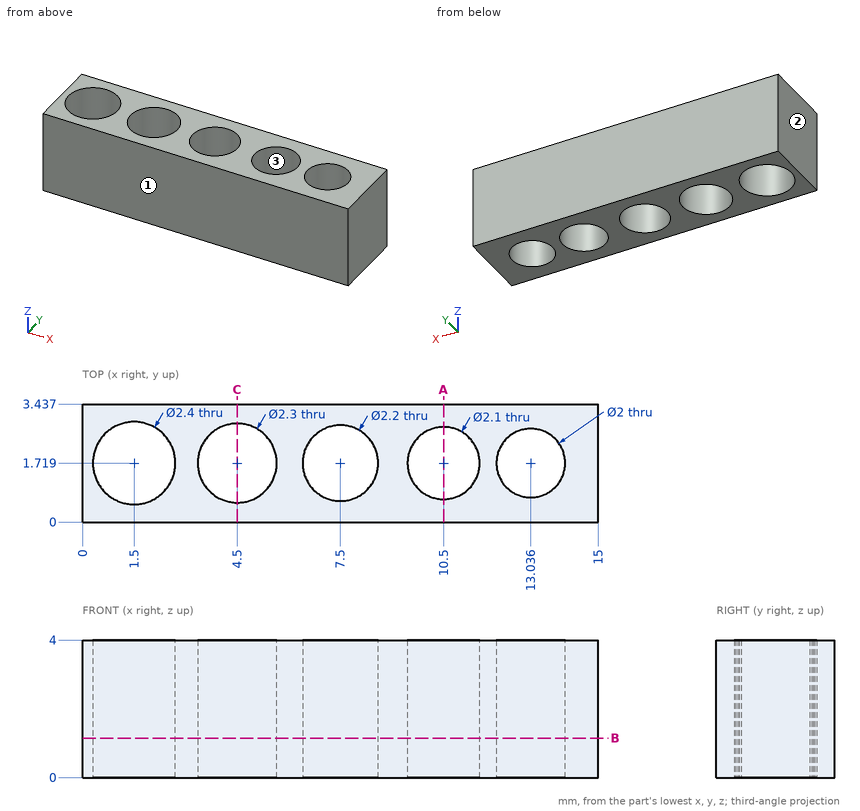
Here's the drawing with two shaded views (mm, measured from the low corner). I have some questions. Give positions to 0.01 mm unless a question says otherwise; leave off trailing zeros. Order: outer loops, then holes, each group sorted by start corner. A loop starts at its lowest first (then second) coordinate and runs counter-clockwise, first axis right, second up. Notation, with made-up numbers: (70.25, 21) -> (109.25, 21) arc R20 ccw to (109.25, 53) -> close; hole circle Ø11 at (89, 6.25). An arc over 180 degrees is marked (long way). Use a Markdown table: item, result. Add a question column.
Item 1: Imagine slicing it at A-A on x = 10.5. Please give me the cut outline in (y, z).
Item 2: Imagine slicing it at C-C on x = 4.5. Please give me the cut outline in (y, z).
Item 3: I need wall thicknesses on line 1 (Y direction, x = 7.5, z = 1.5); line 2 (X direction, y = 1.1, z = 2.95); line 3 (Y direction, x = 4.5, z = 2.85). Which ranges of each line are inside material? Lowest first, please.
Item 4: If we mould it in two halves opening along Y, with no side actions, what happens to the marked faces 1, 2 and 3? For each: pulls with the +Y half, pulls with the -Y half, needs draft (parallel to the pull), parting line crosses it, or undercut.
Item 5: Will this pin go through, and if not, where does the flat tip stop? pin 1 (2 mm diameter, centred on x = 7.5, y = 1, fed in from -Z).
Item 6: Imagine slicing it at B-B on z = 1.15. Please give me the cut outline in (x, y).
Data:
| question | item | result |
|---|---|---|
| 1 | outline | (0, 0) -> (0.67, 0) -> (0.67, 4) -> (0, 4) -> close; (2.77, 0) -> (3.44, 0) -> (3.44, 4) -> (2.77, 4) -> close |
| 2 | outline | (0, 0) -> (0.57, 0) -> (0.57, 4) -> (0, 4) -> close; (2.87, 0) -> (3.44, 0) -> (3.44, 4) -> (2.87, 4) -> close |
| 3 | line 1 | y = 0 to 0.62, 2.82 to 3.44 |
| 3 | line 2 | x = 0 to 0.47, 2.53 to 3.53, 5.47 to 6.59, 8.41 to 9.65, 11.35 to 12.25, 13.82 to 15 |
| 3 | line 3 | y = 0 to 0.57, 2.87 to 3.44 |
| 4 | face 1 | pulls with the -Y half |
| 4 | face 2 | needs draft |
| 4 | face 3 | undercut |
| 5 | pin 1 | stops at z = 0 |
| 6 | outline | (0, 0) -> (15, 0) -> (15, 3.44) -> (0, 3.44) -> close; hole circle Ø2.4 at (1.5, 1.72); hole circle Ø2.3 at (4.5, 1.72); hole circle Ø2.2 at (7.5, 1.72); hole circle Ø2.1 at (10.5, 1.72); hole circle Ø2 at (13.04, 1.72) |
